Drawing for the job (mm, zero at the part's lowest x, y, z). Coordinates: 2 decimals unless noted, no trailing zeros. Order: outer loops, then holes, each group sorted by start corner. A loop starts at its lowest first (then second) coordinate and runs counter-clockwise, first axis right, second up.
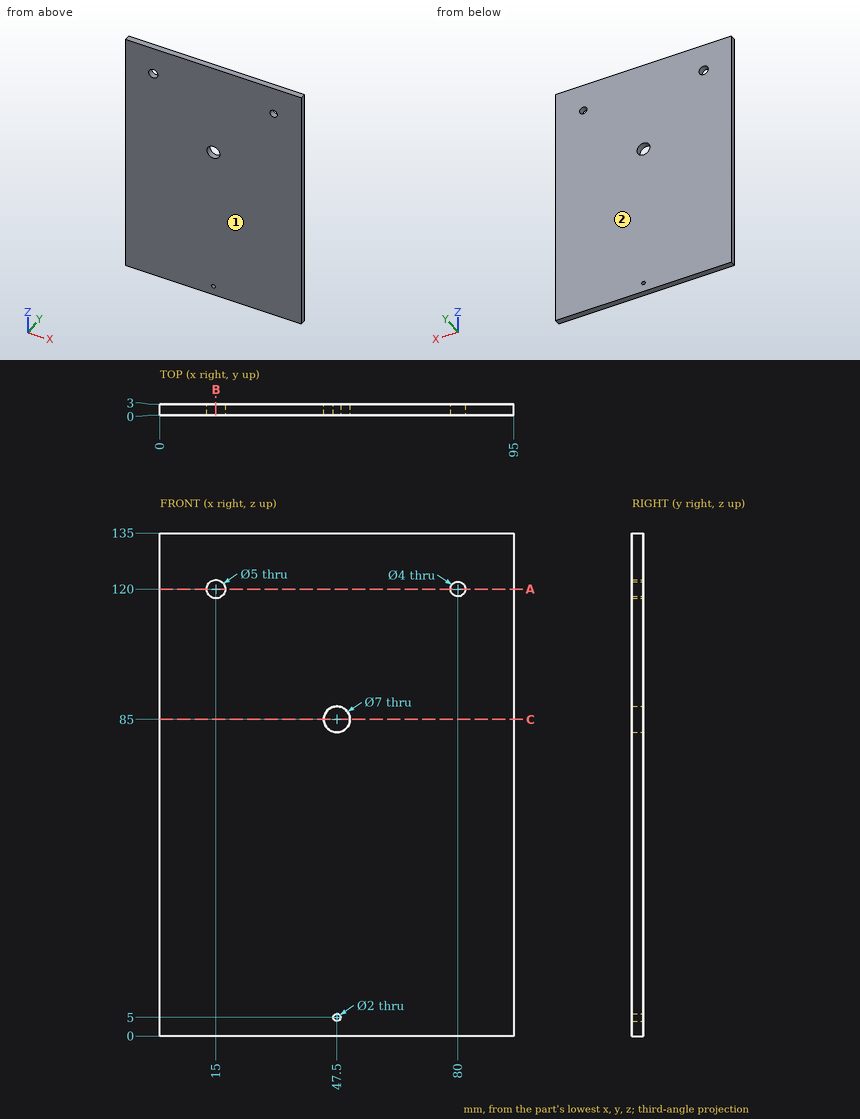
(1) Drop a flat-ended pin along its axis: pin 1 (4.5 mm diameter, centred on x = 15, z = 120, fed in from -Y). Give the stop position or say it passes through.
(2) Slice it at C-C, the plane z = 85. Give the cut face in (x, y).
(3) Pull direction Y, two halves, no side cores. Call the marked faces 1 and 2: +Y half, -Y half, draft (parallel to the pull), parting line (faces both ways), or undercut.
(4) Slice it at A-A, the plane z = 120. Give the cut face in (x, y), then the cut area to 3 significant figures.
(5) Slice it at B-B, the plane x = 15. Give the cut face in (y, z).
(6) Probe line 1 (X direction, y = 2.35, z = 120); line 2 (X direction, y = 2, z = 85); line 3 (Z direction, x = 47.5, y = 2.4). List the from-to ranges inside material, lowest first.
Here are the results:
1. pin 1: passes through
2. outline: (0, 0) - (44, 0) - (44, 3) - (0, 3) - close; (51, 0) - (95, 0) - (95, 3) - (51, 3) - close
3. face 1: -Y half
3. face 2: +Y half
4. outline: (0, 0) - (12.5, 0) - (12.5, 3) - (0, 3) - close; (17.5, 0) - (78, 0) - (78, 3) - (17.5, 3) - close; (82, 0) - (95, 0) - (95, 3) - (82, 3) - close
4. area: 258 mm2
5. outline: (0, 0) - (3, 0) - (3, 117.5) - (0, 117.5) - close; (0, 122.5) - (3, 122.5) - (3, 135) - (0, 135) - close
6. line 1: x = 0 to 12.5, 17.5 to 78, 82 to 95
6. line 2: x = 0 to 44, 51 to 95
6. line 3: z = 0 to 4, 6 to 81.5, 88.5 to 135
